Can you work these out from the model? Positions are in its coordinate system, mm. A direction names the side the tool comes from. Coordinates: 2 decimals unless noted, no trailing zeros. Loops run counter-clockwise (first coordinate to the right, second up) from the corner with the lowest first, then second, coordinate; pieces in that order, holes last.
```python
from build123d import *

# Parameters (mm, degrees)
BOSS_EXTRUDE1_DEPTH      = 36
BOSS_EXTRUDE1_DEPTH_BACK = 36
SKETCH1_R                = 30
SKETCH1_R_2              = 18.065
BOSS_EXTRUDE2_DEPTH      = 4
BOSS_EXTRUDE2_DEPTH_BACK = 4
SKETCH1_3_R              = 62
SKETCH1_3_R_2            = 30
BOSS_EXTRUDE3_DEPTH      = 25
BOSS_EXTRUDE3_DEPTH_BACK = 25
SKETCH1_4_R              = 70
SKETCH1_4_R_2            = 62


with BuildPart() as part:
    # Sketch1 → Boss-Extrude1 (new, two sides: drawn at the far end of the back side and taken through both)
    with BuildSketch(Plane.XY.offset(-BOSS_EXTRUDE1_DEPTH_BACK)):
        Circle(SKETCH1_R)
        Circle(SKETCH1_R_2, mode=Mode.SUBTRACT)
    extrude(amount=BOSS_EXTRUDE1_DEPTH + BOSS_EXTRUDE1_DEPTH_BACK)

    # Sketch1<3> → Boss-Extrude2 (add, two sides: drawn at the far end of the back side and taken through both)
    with BuildSketch(Plane.XY.offset(-BOSS_EXTRUDE2_DEPTH_BACK)):
        Circle(SKETCH1_3_R)
        Circle(SKETCH1_3_R_2, mode=Mode.SUBTRACT)
    extrude(amount=BOSS_EXTRUDE2_DEPTH + BOSS_EXTRUDE2_DEPTH_BACK)

    # Sketch1<4> → Boss-Extrude3 (add, two sides: drawn at the far end of the back side and taken through both)
    with BuildSketch(Plane.XY.offset(-BOSS_EXTRUDE3_DEPTH_BACK)):
        Circle(SKETCH1_4_R)
        Circle(SKETCH1_4_R_2, mode=Mode.SUBTRACT)
    extrude(amount=BOSS_EXTRUDE3_DEPTH + BOSS_EXTRUDE3_DEPTH_BACK)


solid = part.part
```
Item 1: Suppose I cut it at A-A, the plane x = 0. Please give me the cut outline in (y, z) (3 decimals), plus the area to 3 significant figures.
Results are:
outline: (-70, -25) - (-62, -25) - (-62, -4) - (-30, -4) - (-30, -36) - (-18.065, -36) - (-18.065, 36) - (-30, 36) - (-30, 4) - (-62, 4) - (-62, 25) - (-70, 25) - close; (18.065, -36) - (30, -36) - (30, -4) - (62, -4) - (62, -25) - (70, -25) - (70, 25) - (62, 25) - (62, 4) - (30, 4) - (30, 36) - (18.065, 36) - close
area: 3,030 mm2
Item 2: I'm going to push flat-ended pins straight in: P1, Ø1.5, axis at x = -50.5, z = 18.5, coming from the +Y side; P2, Ø6, axis at y = -5, z = 25, coming from the -X side; P3, Ø3, axis at x = -49.5, y = 16, coming from the +Z side. Where does each tip first touch, or does it pass through?
Results are:
P1: stops at y = 49.24
P2: stops at x = -69.97
P3: stops at z = 4
Item 3: On a 3-axis mill with a long thin cutter (end or side, diameter ignored), from which of +Z, -Z, +X, -X, +Y, -Y can I reach the whole of each face in a straight line? I mean faces 4 (the face through (-15, -27, -4)), 5 (the face through (-6, -62, 25)), 6 (the face through (-3.916, -17.635, -0.504)). Say none if no direction works.
Results are:
face 4: -Z
face 5: +Z
face 6: +Z, -Z
Item 4: We'd pull the mould along X, two halves only. Please class faces 1 (the face through (-6, -62, -25)), 2 (the face through (-15, -27, 4)), 3 (the face through (-55.55, -42.594, -0.35)): +X half, -X half, draft (parallel to the pull), parting line (faces both ways), or undercut.
Results are:
face 1: draft
face 2: undercut
face 3: parting line
Item 5: I need wall thicknesses on line 1 along Y through (x, z) = (0, -6) (3 decimals); line 2 along X through (y, z) = (2, -12); line 3 along Y through (x, z) = (23.5, -15). Which ranges of each line are inside material? Lowest first, please.
Results are:
line 1: y = -70 to -62, -30 to -18.065, 18.065 to 30, 62 to 70
line 2: x = -69.97 to -61.97, -29.93 to -17.95, 17.95 to 29.93, 61.97 to 69.97
line 3: y = -65.94 to -57.37, -18.65 to 18.65, 57.37 to 65.94
Item 6: Suppose I cut it at D-D, the plane x = 50.5. Please give me the cut outline in (y, z), plus the area to 3 significant figures.
Results are:
outline: (-48.47, -25) - (-35.97, -25) - (-35.97, -4) - (35.97, -4) - (35.97, -25) - (48.47, -25) - (48.47, 25) - (35.97, 25) - (35.97, 4) - (-35.97, 4) - (-35.97, 25) - (-48.47, 25) - close
area: 1,830 mm2
Item 7: Suppose I cut it at C-C, the plane z = -7.5. Please give me the cut outline in (x, y) (3 decimals), plus the area to 3 significant figures.
Results are:
outline: circle Ø140 at (0, 0); circle Ø60 at (0, 0); hole circle Ø124 at (0, 0); hole circle Ø36.13 at (0, 0)
area: 5,120 mm2
